Can you work these out from the model? Positions are in its coordinate system, mm. A direction names the side the tool comes from. Coordinates: 2 decimals unless noted, no trailing zeros. Order: outer loops, then holes, each group sorted by start corner. A loop starts at its lowest first (then second) coordinate and runs counter-clockwise, first axis right, second up. Notation, with made-up numbers: (37, 15.25) -> (72, 15.25) arc R29 cw to (72, 35.25) -> close; hole circle Ø8 at (41.25, -28). An arc over 180 degrees is marked (long way). Answer in a Markdown table with one row per item.
Autodesk Inventor part; units mm, degrees
ref_plane "YZ Plane" through (0, 0, 0) normal (1, 0, 0) x (0, 1, 0)
ref_plane "XZ Plane" through (0, 0, 0) normal (0, 1, 0) x (-1, 0, 0)
ref_plane "XY Plane" through (0, 0, 0) normal (0, 0, 1) x (1, 0, 0)
sketch "Sketch1" plane through (0, 0, 0) normal (0, 1, 0) x (-1, 0, 0)
  line L0 (2, 0) -> (53, 0)
  line L1 (58, -36) -> (2, -36)
  line L2 (0, -34) -> (0, -2)
  line L3 (60, -34) -> (60, -29)
  line L4 (58, -27) -> (55, -27)
  line L5 (55, -27) -> (55, -2)
  arc A0 (58, -36) -> (60, -34) centre (58, -34) ccw
  arc A1 (0, -34) -> (2, -36) centre (2, -34) ccw
  arc A2 (55, -2) -> (53, 0) centre (53, -2) ccw
  arc A3 (2, 0) -> (0, -2) centre (2, -2) ccw
  arc A4 (60, -29) -> (58, -27) centre (58, -29) ccw
  point P0 (0, 0)
  point P1 (60, -36)
  point P2 (55, 0)
  point P3 (0, -36)
  point P4 (60, -27)
  dimension "d0" = 60
  dimension "d47" = 36
  dimension "d48" = 9
  dimension "d49" = 5
  dimension "d68" = 2
  dimension "d87" = 2
extrude "Extrusion1" add sketch "Sketch1" along normal blind 3
sketch "Sketch7" plane through (0, 3, 0) normal (0, 1, 0) x (1, 0, 0)
  line L0 (-53, 0) -> (-2, 0)
  line L1 (0, 2) -> (0, 34)
  line L2 (-2, 36) -> (-58, 36)
  line L3 (-56.25, 31.5) -> (-3.75, 31.5)
  line L4 (-3.75, 31.5) -> (-3.75, 4.5)
  line L5 (-3.75, 4.5) -> (-56.25, 4.5)
  line L6 (-56.25, 4.5) -> (-56.25, 31.5)
  line L7 (-55, 27) -> (-55, 2)
  line L8 (-60, 34) -> (-60, 29)
  line L9 (-58, 27) -> (-55, 27)
  arc A0 (-55, 2) -> (-53, 0) centre (-53, 2) ccw
  arc A1 (-2, 0) -> (0, 2) centre (-2, 2) ccw
  arc A2 (0, 34) -> (-2, 36) centre (-2, 34) ccw
  arc A3 (-58, 36) -> (-60, 34) centre (-58, 34) ccw
  arc A4 (-60, 29) -> (-58, 27) centre (-58, 29) ccw
  point P0 (-14.75, 4.5)
  dimension "d42" = 27
  dimension "d43" = 52.5
  dimension "d44" = 4.5
  dimension "d45" = 11
  dimension "d50" = 3.75
hole "Hole1" at (-56.25, 3, -31.5) at (-3.75, 3, -31.5) at (-14.75, 3, -4.5) direction (0, -1, 0) diameter 3 depth 10.25
sketch "Sketch8" plane through (0, 3, 0) normal (0, 1, 0) x (1, 0, 0)
  line L0 (-52.75, 33.5) -> (-7.25, 33.5)
  line L1 (-7.25, 24) -> (-52.75, 24)
  circle A0 centre (-56.25, 31.5) radius 1.5
  circle A1 centre (-3.75, 31.5) radius 1.5
  circle A2 centre (-56.25, 31.5) radius 3.5
  circle A3 centre (-3.75, 31.5) radius 3.5
  line L2 (-2, 36) -> (-58, 36)
  line L3 (-54.75, 28.3377) -> (-54.75, 22)
  line L4 (-54.75, 22) -> (-5.25, 22)
  line L5 (-5.25, 35.5) -> (-54.75, 35.5)
  line L6 (-54.75, 35.5) -> (-54.75, 34.6623)
  line L7 (-52.75, 33.5) -> (-53.3777, 33.5)
  line L8 (-52.75, 24) -> (-52.75, 29.5)
  line L9 (-52.75, 29.5) -> (-52.75, 31.5)
  line L10 (-52.75, 33.5) -> (-52.75, 31.5)
  line L11 (-52.75, 29.5) -> (-53.3777, 29.5)
  line L12 (-7.25, 33.5) -> (-7.25, 31.5)
  line L13 (-7.25, 31.5) -> (-7.25, 29.5)
  line L14 (-7.25, 29.5) -> (-7.25, 24)
  line L15 (-7.25, 33.5) -> (-6.6223, 33.5)
  line L16 (-7.25, 29.5) -> (-6.6223, 29.5)
  line L17 (-5.25, 35.5) -> (-5.25, 34.6623)
  line L18 (-5.25, 28.3377) -> (-5.25, 22)
  point P0 (0, 0)
  dimension "d73" = 9.5
  dimension "d74" = 45.5
  dimension "d75" = 7
  dimension "d76" = 7
  dimension "d77" = 2.5
  dimension "d78" = 2
  dimension "d81" = 2
  dimension "d82" = 9.5
  dimension "d83" = 2
  dimension "d85" = 49.5
  dimension "d86" = 49.5
extrude "Extrusion6" add sketch "Sketch8" along normal blind 6 contours L7 A2 L6 L5 L17 A3 L15 L0 | L11 L8 L1 L14 L16 A3 L18 L4 L3 A2
sketch "Sketch9" plane through (0, 3, 0) normal (0, 1, 0) x (1, 0, 0)
  line L0 (-52.75, 29.5) -> (-52.75, 24)
  line L1 (-52.75, 24) -> (-7.25, 24)
  line L2 (-7.25, 24) -> (-7.25, 29.5)
  line L3 (-6.6223, 33.5) -> (-53.3777, 33.5)
  line L4 (-52.75, 29.5) -> (-52.75, 33.5)
  line L5 (-7.25, 29.5) -> (-6.6223, 29.5)
  line L6 (-7.25, 29.5) -> (-7.25, 33.5)
  point P0 (0, 0)
extrude "Extrusion7" cut sketch "Sketch9" against normal up to next
properties part number "MidPlate v2"
(1) Suppose I cut it at B-B (x = -47.5). Please give me the cut outline in (y, z), and give its area (4 significant figures).
Response values:
| item | result |
|---|---|
| outline | (0, -36) -> (3, -36) -> (3, -35.5) -> (9, -35.5) -> (9, -33.5) -> (0, -33.5) -> close; (0, -24) -> (9, -24) -> (9, -22) -> (3, -22) -> (3, 0) -> (0, 0) -> close |
| area | 103.5 mm2 |
(2) Suppose I cut it at D-D (z = -31.5). Please give me the cut outline in (x, y), and give its area (3 significant figures).
Response values:
| item | result |
|---|---|
| outline | (-60, 0) -> (-57.75, 0) -> (-57.75, 3) -> (-60, 3) -> close; (-54.75, 0) -> (-52.75, 0) -> (-52.75, 3) -> (-54.75, 3) -> close; (-7.25, 0) -> (-5.25, 0) -> (-5.25, 3) -> (-7.25, 3) -> close; (-2.25, 0) -> (0, 0) -> (0, 3) -> (-2.25, 3) -> close |
| area | 25.5 mm2 |
(3) Suppose I cut it at A-A (z = -25.5). Please give me the cut outline in (x, y), and give its area (3 significant figures).
Response values:
| item | result |
|---|---|
| outline | (-55, 0) -> (-52.75, 0) -> (-52.75, 9) -> (-54.75, 9) -> (-54.75, 3) -> (-55, 3) -> close; (-7.25, 0) -> (0, 0) -> (0, 3) -> (-5.25, 3) -> (-5.25, 9) -> (-7.25, 9) -> close |
| area | 52.5 mm2 |
(4) We'd pull the mould along X, two halves only. Please class faces 1 (the flat face through (-7.25, 4, -28)), 2 (the flat face through (-55, 1, -15)), 3 (the flat face through (-30, 6, -35.5)): +X half, -X half, draft (parallel to the pull), parting line (faces both ways), or undercut.
Response values:
| item | result |
|---|---|
| face 1 | undercut |
| face 2 | -X half |
| face 3 | draft |
(5) On a 3-axis mill with a long thin cutter (end or side, diameter ignored), from which of +Z, -Z, +X, -X, +Y, -Y can I reach the whole of each face in a straight line? I mean faces 4 (the flat face through (-5.25, 6, -25)), 5 (the flat face through (-30, 5, -24)), 6 (the cylindrical face through (-6, 5.96, -28.82)). Say none if no direction works.
Response values:
| item | result |
|---|---|
| face 4 | +Z, -Z, +X, +Y |
| face 5 | +Y, -Y |
| face 6 | +X, +Y |
(6) I need wall thicknesses on line 1 (X direction, y = 0.8, z = -31.5); line 2 (X direction, y = 1.4, z = -4.5); line 3 (Z direction, x = -14.75, y = 1.7). Which ranges of each line are inside material? Lowest first, please. Write a range as [from, to].
Response values:
| item | result |
|---|---|
| line 1 | [-60, -57.75], [-54.75, -52.75], [-7.25, -5.25], [-2.25, 0] |
| line 2 | [-55, -16.25], [-13.25, 0] |
| line 3 | [-36, -33.5], [-24, -6], [-3, 0] |
(7) Suppose I cut it at C-C (y = 1.25). Please give me the cut outline in (x, z).
Response values:
| item | result |
|---|---|
| outline | (-60, -34) arc R2 ccw to (-58, -36) -> (-2, -36) arc R2 ccw to (0, -34) -> (0, -2) arc R2 ccw to (-2, 0) -> (-53, 0) arc R2 ccw to (-55, -2) -> (-55, -27) -> (-58, -27) arc R2 ccw to (-60, -29) -> close; hole circle Ø3 at (-56.25, -31.5); hole (-52.75, -33.5) -> (-7.25, -33.5) -> (-7.25, -24) -> (-52.75, -24) -> close; hole circle Ø3 at (-14.75, -4.5); hole circle Ø3 at (-3.75, -31.5) |
(8) Will these pins go through, and if not, where does the flat tip stop? pin 1 Ø0.9 at (x, y) = (-56.5, 1) entering from +Z; pin 2 Ø0.7 at (x, y) = (-7, 5.5) entering from -Z; pin 3 Ø5 at (y, z) = (7, -23) entering from +X.
Response values:
| item | result |
|---|---|
| pin 1 | z = -27 |
| pin 2 | z = -35.5 |
| pin 3 | x = -5.25 |
